Verification items for the finished model (mm, model axes). Round coordinates to 2 decimals unless told otherwise and drop trailing zeros. Write each loop counter-clockwise with the first axis right and the second up, starting at its lowest first coordinate (ties: lowest second). Pieces come first, ordered by that corner, then holes. Notation, with made-up numbers: M 72.5,52.25 L 90.5,52.25 A27 ccw 90.5,74.25 Z; hole C 73,-7.75 d9. An arc over 180 degrees is marked long. One line per question, with ' | ' between items.
Autodesk Inventor part; units mm, degrees
ref_plane "YZ Plane" through (0, 0, 0) normal (1, 0, 0) x (0, 1, 0)
ref_plane "XZ Plane" through (0, 0, 0) normal (0, 1, 0) x (-1, 0, 0)
ref_plane "XY Plane" through (0, 0, 0) normal (0, 0, 1) x (1, 0, 0)
sketch "Sketch1" plane through (0, 0, 0) normal (0, 0, 1) x (1, 0, 0)
  line L0 (0, 61.5875) -> (62, 61.5875) construction
  line L1 (62, 61.5875) -> (62, -0.4125) construction
  line L2 (62, -0.4125) -> (0, -0.4125) construction
  line L3 (0, -0.4125) -> (0, 61.5875) construction
  line L4 (48.4322, 11.2012) -> (48.4322, 37.9079)
  line L5 (20.3147, 37.9079) -> (20.3147, 2.4417)
  line L6 (24.0433, 39.9079) -> (22.3147, 39.9079)
  line L7 (46.4322, 39.9079) -> (24.0433, 39.9079)
  arc A0 (22.3147, 39.9079) -> (20.3147, 37.9079) centre (22.3147, 37.9079) ccw
  circle A1 centre (23.179, 26.4983) radius 1.5
  circle A2 centre (45.5157, 37.2749) radius 1.5
  line L8 (16.613, -7.1773) -> (12.7525, -9.2371)
  line L9 (22.9974, 0.5619) -> (47.1149, 9.3214)
  arc A3 (20.3147, 2.4417) -> (22.9974, 0.5619) centre (22.3147, 2.4417) ccw
  arc A4 (47.1149, 9.3214) -> (48.4322, 11.2012) centre (46.4322, 11.2012) ccw
  arc A5 (48.4322, 37.9079) -> (46.4322, 39.9079) centre (46.4322, 37.9079) ccw
  point P0 (0, 0)
  point P1 (48.4322, 39.9079)
  point P2 (48.4322, 9.7998)
  point P3 (20.3147, -0.4125)
  dimension "d9" = 62
  dimension "d18" = 2
  dimension "d19" = 3
  dimension "d20" = 3
  dimension "d27" = 28.1175
  dimension "d47" = 2
extrude "Extrusion2" add sketch "Sketch1" along normal blind 3
sketch "Sketch3" plane through (0, 0, 0) normal (0, 0, -1) x (-1, 0, 0)
  circle A0 centre (-41.0584, 11.8538) radius 4
  circle A1 centre (-27.789, 6.9341) radius 4
  point P0 (0, 0)
  dimension "d51" = 8
  dimension "d52" = 8
extrude "Extrusion4" add sketch "Sketch3" along normal blind 1.5
sketch "Sketch4" plane through (0, 0, 3) normal (0, 0, 1) x (1, 0, 0)
  circle A0 centre (27.789, 6.9341) radius 4
  circle A1 centre (41.0584, 11.8538) radius 4
  circle A2 centre (41.0584, 11.8538) radius 3.25
  circle A3 centre (27.789, 6.9341) radius 3.25
  point P0 (0, 0)
  dimension "d55" = 6.5
  dimension "d56" = 6.5
extrude "Extrusion5" cut sketch "Sketch4" against normal blind 1.5 contours A2 | A3
sketch "Sketch5" plane through (41.0584, 11.8538, 1.5) normal (0, 0, 1) x (1, 0, 0)
  circle A0 centre (-13.2694, -4.9197) radius 3.25
  circle A1 centre (0, 0) radius 3.25
  point P0 (-41.0584, -11.8538)
hole "Hole1" at (27.789, 6.9341, 1.5) at (41.0584, 11.8538, 1.5) direction (0, 0, -1) diameter 3 depth 3 tip angle 118 counterbore diameter 5 counterbore depth 0.85
properties part number "bump_switch_mount"
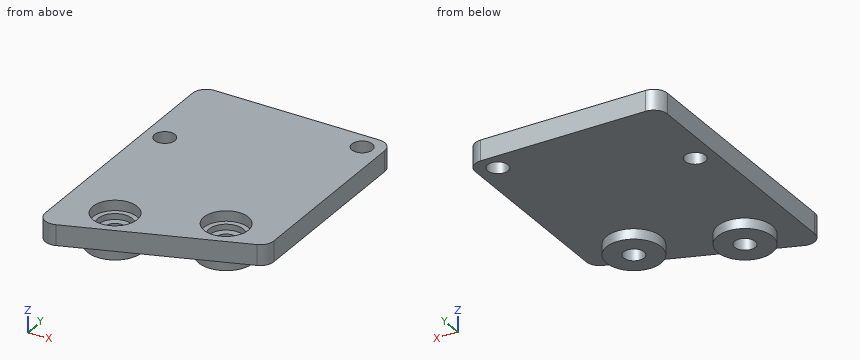
1. Thickness scan on line 1 (Z direction, x = 32.5, y = 33.5); line 2 (X direction, y = 12, z = 1.8); line 3 (Y direction, x = 27, z = 2.7). Record the ranges inside material, lowest first.
Results:
line 1: z = 0 to 3 | line 2: x = 20.31 to 37.81, 44.31 to 48.43 | line 3: y = 2.02 to 3.78, 10.09 to 39.91
2. Section check C-C, the plane z = 2.35. Record the cut outline in (x, y), then the cut area to 3 significant figures.
Results:
outline: M 20.31,2.44 A2 ccw 23,0.56 L 47.11,9.32 A2 ccw 48.43,11.2 L 48.43,37.91 A2 ccw 46.43,39.91 L 22.31,39.91 A2 ccw 20.31,37.91 Z; hole C 23.18,26.5 d3; hole C 27.79,6.93 d6.5; hole C 41.06,11.85 d6.5; hole C 45.52,37.27 d3 | area: 906 mm2
3. Section check B-B, the plane y = 6.5. Record the cut outline in (x, z).
Results:
outline: M 20.31,0 L 23.81,0 L 23.81,-1.5 L 26.35,-1.5 L 26.35,0.65 L 25.33,0.65 L 25.33,1.5 L 24.57,1.5 L 24.57,3 L 20.31,3 Z; M 29.22,-1.5 L 31.77,-1.5 L 31.77,0 L 39.35,0 L 39.35,3 L 31.01,3 L 31.01,1.5 L 30.25,1.5 L 30.25,0.65 L 29.22,0.65 Z
4. Section check D-D, the plane y = 30. Record the cut outline in (x, z).
Results:
outline: M 20.31,0 L 48.43,0 L 48.43,3 L 20.31,3 Z
5. Section check A-A, the plane x = 28.5. Record the cut outline in (y, z).
Results:
outline: M 2.56,0 L 3,0 L 3,-1.5 L 5.61,-1.5 L 5.61,0.65 L 4.54,0.65 L 4.54,1.5 L 3.76,1.5 L 3.76,3 L 2.56,3 Z; M 8.25,-1.5 L 10.87,-1.5 L 10.87,0 L 39.91,0 L 39.91,3 L 10.11,3 L 10.11,1.5 L 9.33,1.5 L 9.33,0.65 L 8.25,0.65 Z
6. Go/stop test with flat-tipped pins: P1, Ø1.5, axis at x = 40, y = 11, coming from the +Z side; P2, Ø1.8, axis at x = 41.06, y = 11.85, coming from the -Z side; P3, Ø3, axis at x = 36.5, y = 30.5, coming from the -Z side; P4, Ø2.5, axis at x = 29, y = 7.5, coming from the +Z side. Record where each tip stops, or that it passes through.
Results:
P1: stops at z = 0.65 | P2: passes through | P3: stops at z = 0 | P4: stops at z = 1.5
